from build123d import *

# Parameters (mm, degrees)
BASE_FLANGE1_DEPTH        = 18.5
FILLET3_RADIUS            = 18.5
FILLET3_LENGTH            = 5.35
FILLET4_RADIUS            = 18.5
FILLET4_LENGTH            = 5.35
CUT_EXTRUDE6_DEPTH        = 57.986840586
CUT_EXTRUDE6_DEPTH_BACK   = 57.986840586
SKETCH23_R                = 10.5
M3X0_5_TAPPED_HOLE1_D     = 2.5
M3X0_5_TAPPED_HOLE1_DEPTH = 5.35
M3X0_5_TAPPED_HOLE2_D     = 2.5


# Sheet-metal steps are written as plain solids
with BuildPart() as part:
    # Sketch20 → Base-Flange1 (new, symmetric)
    with BuildSketch(Plane.XY):
        with BuildLine():
            Line((43, -32.5), (7.730000066, -32.5))
            ThreePointArc((7.730000066, -32.5), (2.264064601, -30.235935399), (0, -24.769999934))
            Line((0, -24.769999934), (0, 24.769999934))
            ThreePointArc((0, 24.769999934), (2.264064601, 30.235935399), (7.730000066, 32.5))
            Line((7.730000066, 32.5), (43, 32.5))
            Line((43, 32.5), (43, 27.15))
            Line((43, 27.15), (7.730000066, 27.15))
            ThreePointArc((7.730000066, 27.15), (6.04708588, 26.45291412), (5.35, 24.769999934))
            Line((5.35, 24.769999934), (5.35, -24.769999934))
            ThreePointArc((5.35, -24.769999934), (6.04708588, -26.45291412), (7.730000066, -27.15))
            Line((7.730000066, -27.15), (43, -27.15))
            Line((43, -27.15), (43, -32.5))
        make_face()
    extrude(amount=BASE_FLANGE1_DEPTH, both=True)

    # Fillet3: full round fillet: the end face becomes a half cylinder, R = half its width
    fillet3_face = Plane((43, 29.825, 0), x_dir=(0, 1, 0), z_dir=(1, 0, 0))  # on the end face: x along it, z out of the body
    fillet3_slab = fillet3_face.offset(-FILLET3_RADIUS / 2) * Box(FILLET3_LENGTH, 2 * FILLET3_RADIUS, FILLET3_RADIUS, mode=Mode.PRIVATE)  # the body's end, R deep
    fillet3_round = Plane((24.5, 29.825, 0), x_dir=(1, 0, 0), z_dir=(0, 1, 0)) * Cylinder(FILLET3_RADIUS, FILLET3_LENGTH, mode=Mode.PRIVATE)  # its axis R under the face
    add(fillet3_slab - fillet3_round, mode=Mode.SUBTRACT)

    # Fillet4: full round fillet: the end face becomes a half cylinder, R = half its width
    fillet4_face = Plane((43, -29.825, 0), x_dir=(0, 1, 0), z_dir=(1, 0, 0))  # on the end face: x along it, z out of the body
    fillet4_slab = fillet4_face.offset(-FILLET4_RADIUS / 2) * Box(FILLET4_LENGTH, 2 * FILLET4_RADIUS, FILLET4_RADIUS, mode=Mode.PRIVATE)  # the body's end, R deep
    fillet4_round = Plane((24.5, -29.825, 0), x_dir=(1, 0, 0), z_dir=(0, 1, 0)) * Cylinder(FILLET4_RADIUS, FILLET4_LENGTH, mode=Mode.PRIVATE)  # its axis R under the face
    add(fillet4_slab - fillet4_round, mode=Mode.SUBTRACT)

    # Sketch23 → Cut-Extrude6 (cut, two sides: drawn at the far end of the back side and taken through both)
    with BuildSketch(Plane(origin=(0, 0, 0), x_dir=(1, 0, 0), z_dir=(0, 1, 0)).offset(-CUT_EXTRUDE6_DEPTH_BACK)):
        with Locations(Location((24.5, 0, 0), (0, 0, 270))):
            Circle(SKETCH23_R)
    extrude(amount=CUT_EXTRUDE6_DEPTH + CUT_EXTRUDE6_DEPTH_BACK, mode=Mode.SUBTRACT)

    # M3x0.5 Tapped Hole1
    with Locations(Plane(origin=(0, 32.5, 0), x_dir=(1, 0, 0), z_dir=(0, 1, 0))):
        with Locations((38.127028289, 3.21), (10.882456169, -3.25)):
            Hole(M3X0_5_TAPPED_HOLE1_D / 2, depth=M3X0_5_TAPPED_HOLE1_DEPTH)

    # M3x0.5 Tapped Hole2 (through all)
    with Locations(Plane(origin=(0, -32.5, 0), x_dir=(-1, 0, 0), z_dir=(0, -1, 0))):
        with Locations((-10.882456169, -3.25), (-38.127028289, 3.21)):
            Hole(M3X0_5_TAPPED_HOLE2_D / 2)


solid = part.part
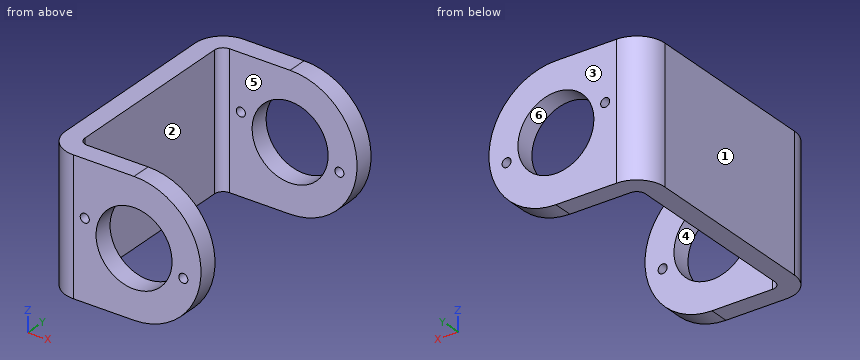
Source: CAD feature listing. Evaluate the final solid. Frame: model axes, mm. Face numbers are marked on the shaded views. A direction names the side the tool comes from. Round coordinates to 2 decimals unless told otherwise and drop trailing zeros. Loops run counter-clockwise (first coordinate to the right, second up) from the corner with the lowest first, then second, coordinate; pieces in that order, holes last. Notation, with made-up numbers: (86.25, -29.75) - (135.25, -29.75) arc R4 cw to (135.25, -24.75) - close; hole circle Ø9 at (-4, -37.5). An arc over 180 degrees is marked (long way). Write item = value, one per line. Start each with the question number.
Item 1: Material intervals for line 1 (Y direction, x = 34, z = 13.5); line 2 (X direction, y = -28, z = 3); line 3 (Y direction, x = 7.5, z = -8.5), sorted ascending.
Item 2: Section query B-B on x = 30. Output: boundary loops of the cut face in (y, z).
Item 3: Section query C-C on y = 12.5. Output: boundary loops of the cut face in (x, z), plus the area to 3 significant figures.
Item 4: First-contact query: pin 1 Ø4 at (y, z) = (18.5, 13.5) entering from +X; pin 2 Ø3 at (x, z) = (38.13, -3.21) entering from +Y. Flat tips, straight axial feed; report the tip coordinate or a pass-through.
Item 5: Mould query, pull axis X, two halves, no side actions, for the marked faces 1, 2, 3 and 4. Classes: released by +X, released by -X, zero draft, split by the parting line, or undercut.
Item 6: Section query A-A on z = 0. Output: boundary loops of the cut face in (x, y), plus the area to 3 significant figures.
Item 7: Reachability of the marked faces 5 and 6 from +Z, -Z, +X, -X, +Y, -Y: full face, straight path, thin tool, end or side. Return the list, or none.
Item 8: Section query D-D on z = -15.5. Output: boundary loops of the cut face in (x, y), plus the area to 3 significant figures.
Results list:
q1.line_1 = -32.5 to -27.15, 27.15 to 32.5
q1.line_2 = 0.71 to 9.66, 12.11 to 14.44, 34.56 to 42.76
q1.line_3 = -32.5 to -27.14, 27.14 to 32.5
q2.outline = (-32.5, -17.66) - (-27.15, -17.66) - (-27.15, -8.94) - (-32.5, -8.94) - close; (-32.5, 8.94) - (-27.15, 8.94) - (-27.15, 17.66) - (-32.5, 17.66) - close; (27.15, -17.66) - (32.5, -17.66) - (32.5, -8.94) - (27.15, -8.94) - close; (27.15, 8.94) - (32.5, 8.94) - (32.5, 17.66) - (27.15, 17.66) - close
q3.outline = (0, -18.5) - (5.35, -18.5) - (5.35, 18.5) - (0, 18.5) - close
q3.area = 198 mm²
q4.pin_1 = 5.35
q4.pin_2 = 32.5
q5.face_1 = released by -X
q5.face_2 = released by +X
q5.face_3 = zero draft
q5.face_4 = undercut
q6.outline = (0, -24.77) arc R7.73 ccw to (7.73, -32.5) - (14, -32.5) - (14, -27.15) - (7.73, -27.15) arc R2.38 cw to (5.35, -24.77) - (5.35, 24.77) arc R2.38 cw to (7.73, 27.15) - (14, 27.15) - (14, 32.5) - (7.73, 32.5) arc R7.73 ccw to (0, 24.77) - close; (35, -32.5) - (43, -32.5) - (43, -27.15) - (35, -27.15) - close; (35, 27.15) - (43, 27.15) - (43, 32.5) - (35, 32.5) - close
q6.area = 503 mm²
q7.face_5 = +Z, -Z, +X
q7.face_6 = +Y, -Y
q8.outline = (0, -24.77) arc R7.73 ccw to (7.73, -32.5) - (34.6, -32.5) - (34.6, -27.15) - (7.73, -27.15) arc R2.38 cw to (5.35, -24.77) - (5.35, 24.77) arc R2.38 cw to (7.73, 27.15) - (34.6, 27.15) - (34.6, 32.5) - (7.73, 32.5) arc R7.73 ccw to (0, 24.77) - close
q8.area = 638 mm²
